Build history of the part. All positions in model axes, mm. A direction names the side the tool comes from. Give positions to 0.01 mm unless a question says otherwise; leave off trailing zeros. Write each loop counter-clockwise with the first axis right and the second up, starting at its lowest first coordinate (ties: lowest second). Pieces come first, ordered by that corner, then holes. Notation, with made-up numbers: M -7,20 L 5,20 A30 cw 5,45 Z; hole C 19,13 d4. An arc over 180 degrees is marked long. Return JSON: item names as keys, results as strings. Group by question number.
Q1. Wall check: probe 1 along Y at (x, z) = (0, 2); probe 2 along Y at (x, z) = (3.25, 14); probe 3 along X at (y, z) = (2.5, 9.5). Give the ranges that are in metal, low to high.
Q2. Flat gauge pins, fed straight in: pin 1 Ø1.5 at (x, y) = (0, 0) entering from -Z; pin 2 Ø1.5 at (y, z) = (2.5, 5.5) entering from -X. Where does each tip first touch, or does it go through?
Q3. Band-saw the part on B-B, the plane y = -2.75. Give the cut face in (x, z).
Q4. Band-saw the part on A-A, the plane z = 13.75. Give the cut face in (x, y), then the cut area to 3 significant figures.
Q5. Tool access for faces 1 (the conical face through (-0.05, -0.21, 19.48)), 2 (the cylindrical face through (-0.27, -1.22, 1.98)): list every direction of +Z, -Z, +X, -X, +Y, -Y with a clear straight run to the whole face (end or side of a thin tool).
Q6. Band-saw the part on C-C, the plane x = -3.5. Give the cut face in (y, z), then the cut area to 3 significant figures.
Q7. Pull direction X, two halves, no side cores. Call faces 3 (the flat face through (0, 3.5, 12)), 4 (the cylindrical face through (0.27, -1.22, 22.02)), 5 (the flat face through (-3, 1.8, 11.8)): +X half, -X half, draft (parallel to the pull), parting line (faces both ways), or undercut.
from build123d import *

# Parameters (mm, degrees)
EXTRUDE_1_DEPTH        = 24
HOLE_WIZARD_M3_1_D     = 2.5
HOLE_WIZARD_M3_1_DEPTH = 3.9
HOLE_WIZARD_M3_1_TIP   = 0.751075774
HOLE_WIZARD_M3_2_D     = 2.5
HOLE_WIZARD_M3_2_DEPTH = 3.9
HOLE_WIZARD_M3_2_TIP   = 0.751075774


with BuildPart() as part:
    # 草图1 → 凸台-拉伸1 (new body)
    with BuildSketch(Plane.XY):
        Polygon((4.041451884, 0), (2.020725942, 3.5), (-2.020725942, 3.5), (-4.041451884, 0), (-2.020725942, -3.5), (2.020725942, -3.5), align=None)
    extrude(amount=EXTRUDE_1_DEPTH)

    # M3 螺纹孔1
    with Locations(Plane(origin=(0, 0, 0), x_dir=(-1, 0, 0), z_dir=(0, 0, -1))):
        with Locations((0, 0)):
            Hole(HOLE_WIZARD_M3_1_D / 2, depth=HOLE_WIZARD_M3_1_DEPTH)
            with Locations((0, 0, -(HOLE_WIZARD_M3_1_DEPTH + HOLE_WIZARD_M3_1_TIP / 2))):  # 118° drill point
                Cone(0, HOLE_WIZARD_M3_1_D / 2, HOLE_WIZARD_M3_1_TIP, mode=Mode.SUBTRACT)

    # M3 螺纹孔2
    with Locations(Plane.XY.offset(24)):
        with Locations((0, 0)):
            Hole(HOLE_WIZARD_M3_2_D / 2, depth=HOLE_WIZARD_M3_2_DEPTH)
            with Locations((0, 0, -(HOLE_WIZARD_M3_2_DEPTH + HOLE_WIZARD_M3_2_TIP / 2))):  # 118° drill point
                Cone(0, HOLE_WIZARD_M3_2_D / 2, HOLE_WIZARD_M3_2_TIP, mode=Mode.SUBTRACT)


solid = part.part
From the geometry:
{
 "1": {"probe 1": "y = -3.5 to -1.25, 1.25 to 3.5", "probe 2": "y = -1.37 to 1.37", "probe 3": "x = -2.6 to 2.6"},
 "2": {"pin 1": "stops at z = 4.2", "pin 2": "stops at x = -3.03"},
 "3": {"outline": "M -2.45,0 L 2.45,0 L 2.45,24 L -2.45,24 Z"},
 "4": {"outline": "M -4.04,0 L -2.02,-3.5 L 2.02,-3.5 L 4.04,0 L 2.02,3.5 L -2.02,3.5 Z", "area": "42.4 mm^2"},
 "5": {"face 1": "+Z", "face 2": "-Z"},
 "6": {"outline": "M -0.94,0 L 0.94,0 L 0.94,24 L -0.94,24 Z", "area": "45.0 mm^2"},
 "7": {"face 3": "draft", "face 4": "undercut", "face 5": "-X half"}
}
